```python
from build123d import *

# Parameters (mm, degrees)
BOSS_EXTRUDE1_DEPTH = 90
SKETCH2_R           = 97.5
CUT_EXTRUDE1_DEPTH  = 72.91
CUT_EXTRUDE10_DEPTH = 72.91
SKETCH13_R          = 3.4
CUT_EXTRUDE13_DEPTH = 17.09


with BuildPart() as part:
    # Sketch1 → Boss-Extrude1 (new body)
    with BuildSketch(Plane(origin=(0, 0, 0), x_dir=(0, 1, 0), z_dir=(0, 0, 1))):
        with BuildLine():
            ThreePointArc((0, 115), (-115, 0), (0, -115))
            add(Edge.make_bspline(
                [(0, -115), (150, -65), (300, -115)],
                knots=[0, 0, 0, 1, 1, 1], degree=2))
            ThreePointArc((300, -115), (415, 0), (300, 115))
            add(Edge.make_bspline(
                [(0, 115), (150, 65), (300, 115)],
                knots=[0, 0, 0, 1, 1, 1], degree=2))
        make_face()
    extrude(amount=BOSS_EXTRUDE1_DEPTH)

    # Sketch2 → Cut-Extrude1 (cut)
    with BuildSketch(Plane(origin=(0, 0, 0), x_dir=(1, 0, 0), z_dir=(0, 0, -1))):
        with Locations(Location((0, 0, 0), (0, 0, 180))):
            Circle(SKETCH2_R)
    extrude(amount=-CUT_EXTRUDE1_DEPTH, mode=Mode.SUBTRACT)

    # Sketch10 → Cut-Extrude10 (cut)
    with BuildSketch(Plane(origin=(0, 0, 0), x_dir=(1, 0, 0), z_dir=(0, 0, -1))):
        with BuildLine():
            ThreePointArc((115, 0), (0, 115), (-115, 0))
            add(Edge.make_bspline(
                [(-92.945702649, -98.510851787), (-98.581524702, -49.255425893), (-115, 0)],
                knots=[0, 0, 0, 1, 1, 1], degree=2))
            ThreePointArc((-92.945702649, -98.510851787), (0, -122.154138558), (92.945702649, -98.510851787))
            add(Edge.make_bspline(
                [(115, 0), (98.581524702, -49.255425893), (92.945702649, -98.510851787)],
                knots=[0, 0, 0, 1, 1, 1], degree=2))
        make_face()
    extrude(amount=-CUT_EXTRUDE10_DEPTH, mode=Mode.SUBTRACT)

    # Sketch13 → Cut-Extrude13 (cut)
    with BuildSketch(Plane(origin=(0, 0, 72.91), x_dir=(1, 0, 0), z_dir=(0, 0, -1))):
        with Locations(Location((0, 20, 0), (0, 0, 180))):
            Circle(SKETCH13_R)
        with Locations(Location((-17.320508076, -10, 0), (0, 0, 180))):
            Circle(SKETCH13_R)
        with Locations(Location((17.320508076, -10, 0), (0, 0, 180))):
            Circle(SKETCH13_R)
    extrude(amount=-CUT_EXTRUDE13_DEPTH, mode=Mode.SUBTRACT)


solid = part.part
```
Work out the finished part from the listing and answer in its coordinate system (mm). Give positions to 0.01 mm unless a question says otherwise; leave off trailing zeros. Loops run counter-clockwise (first coordinate to the right, second up) from the corner with the lowest first, then second, coordinate; pieces in that order, holes last. Notation, with made-up numbers: M 3,13 L 62,13 A10 cw 62,18 Z; hole C 1.5,47 d5. An arc over 180 degrees is marked long. One line per item, written item: value. Start each with the question number.
1. Each of these flat-tipped pins is pushed along its axis until it touches: P1, Ø3, axis at x = 21, z = 45, coming from the -Y side; P2, Ø1, axis at x = 25.5, z = 64, coming from the -Y side; P3, Ø2, axis at x = 88, z = 17.5, coming from the +Y side. Where does it stop, or does it pass through?
2. Find section B-B (y = 339.5). Give the vertices of the cut face in (x, z), and give its area (3 significant figures).
3. Find the intervals of material crossed by probe 1 along Y at (x, z) = (0, 82); probe 2 along Y at (x, z) = (-0.5, 59); probe 3 along Z at (x, y) = (-96, -35), in increasing order.
4. Find section A-A (x = 29). Give the vertices of the cut face in (y, z), and give its area (3 significant figures).
5. Determine the mould class of faces 1 (the face through (-1.36, 122.15, 35.94)), 2 (the face through (-2, 255, 0)), 3 (the face through (2.529, 414.972, 44.37)) for opening direction X: released by +X, released by -X, zero draft, split by the parting line, or undercut.
Reported:
1. P1: stops at y = 120.85
1. P2: stops at y = 120.41
1. P3: stops at y = 375.21
2. outline: M -108,0 L 108,0 L 108,90 L -108,90 Z
2. area: 19,400 mm²
3. probe 1: y = -115 to -23.4, -16.6 to 415
3. probe 2: y = 122.15 to 415
3. probe 3: z = 72.91 to 90
4. outline: M -111.28,72.91 L 119.98,72.91 L 119.98,0 L 411.28,0 L 411.28,90 L -111.28,90 Z
4. area: 30,200 mm²
5. face 1: undercut
5. face 2: zero draft
5. face 3: split by the parting line
